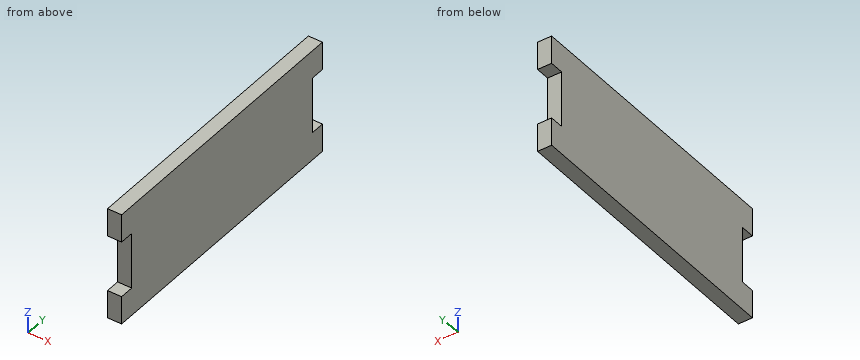
from build123d import *

# Parameters (mm, degrees)
F0_W     = 6.35
F0_H     = 6.35
F1_DEPTH = 6.35


with BuildPart() as f1:
    # F0 (on Right) → F1 (new body)
    with BuildSketch(Plane.YZ):
        with Locations((60.325, 22.225)):
            Rectangle(F0_W, F0_H)
        Polygon((57.15, 19.05), (57.15, 25.4), (-57.15, 25.4), (-57.15, 19.05), (-57.15, 12.7), (-57.15, -12.7), (-57.15, -19.05), (-57.15, -25.4), (57.15, -25.4), (57.15, -19.05), (57.15, -12.7), (57.15, 12.7), align=None)
        with Locations((60.325, 15.875)):
            Rectangle(F0_W, F0_H)
        with Locations((-60.325, 22.225)):
            Rectangle(F0_W, F0_H)
        with Locations((-60.325, 15.875)):
            Rectangle(F0_W, F0_H)
        with Locations((60.325, -15.875)):
            Rectangle(F0_W, F0_H)
        with Locations((-60.325, -15.875)):
            Rectangle(F0_W, F0_H)
        with Locations((60.325, -22.225)):
            Rectangle(F0_W, F0_H)
        with Locations((-60.325, -22.225)):
            Rectangle(F0_W, F0_H)
    extrude(amount=-F1_DEPTH)


solid = f1.part
Here's how the part is built. I have some questions about the finished solid (model axes, mm). Coordinates: 2 decimals unless noted, no trailing zeros. Write each loop counter-clockwise with the first axis right and the second up, starting at its lowest first coordinate (ties: lowest second). Pieces come first, ordered by that corner, then holes.
1) If we section it at B-B (z = 6): List the corners of the cut face in (x, y) for me.
Filled in:
outline: (-6.35, -57.15) - (0, -57.15) - (0, 57.15) - (-6.35, 57.15) - close
2) I'm going to push a flat-ended pin straight in: pin 1 (1 mm diameter, centred on x = -4, z = -2.5, fed in from +Y). Where does the tip first touch, or does it pass through?
Filled in:
pin 1: stops at y = 57.15
3) If I drill on line 1 (Y direction, x = -3, z = 2.5), over which ranges is the centre line in solid material (lowest first)?
Filled in:
line 1: y = -57.15 to 57.15
4) If we section it at A-A (x = -2.5): List the corners of the cut face in (y, z) for me, plus the area to 3 significant figures.
Filled in:
outline: (-63.5, -25.4) - (63.5, -25.4) - (63.5, -12.7) - (57.15, -12.7) - (57.15, 12.7) - (63.5, 12.7) - (63.5, 25.4) - (-63.5, 25.4) - (-63.5, 12.7) - (-57.15, 12.7) - (-57.15, -12.7) - (-63.5, -12.7) - close
area: 6,130 mm2
